from build123d import *

# Parameters (mm, degrees)
BASPROSKE_W         = 15
BASPROSKE_H         = 33
TOOTHCUT_DEPTH      = 50.020403915
TEETHCUTS_COUNT     = 20
TEETHCUTS_ANGLE     = 342
BORSKE_R            = 2
BORE_DEPTH          = 50.0000508
SKETCH1_W           = 29.7
SKETCH1_H           = 29.7
BOSS_EXTRUDE1_DEPTH = 20
SKETCH2_R           = 7.65
CUT_EXTRUDE1_DEPTH  = 35
FILLET2_R           = 1


with BuildPart() as part:
    # BasProSke → Base-Revolve (revolve)
    with BuildSketch(Plane(origin=(0, 0, 0), x_dir=(1, 0, 0), z_dir=(0, 1, 0)), mode=Mode.PRIVATE) as base_revolve_sk:
        with Locations((7.5, 16.5)):
            Rectangle(BASPROSKE_W, BASPROSKE_H)
    revolve(base_revolve_sk.sketch.rotate(Axis((-10, 0, 0), (1, 0, 0)), 180), axis=Axis((-10, 0, 0), (1, 0, 0)))

    # TooCutSke → ToothCut (cut, through all)
    with BuildSketch(Plane(origin=(0, 0, 0), x_dir=(0, 0, -1), z_dir=(1, 0, 0))):
        with BuildLine():
            ThreePointArc((1.489278925, 26.206717637), (0, 26.249), (-1.489278925, 26.206717637))
            ThreePointArc((-1.489278925, 26.206717637), (-2.448651415, 29.690511169), (-4.401620335, 32.730762038))
            ThreePointArc((-4.401620335, 32.730762038), (0, 33.0254), (4.401620335, 32.730762038))
            ThreePointArc((4.401620335, 32.730762038), (2.448651415, 29.690511169), (1.489278925, 26.206717637))
        make_face()
    toothcut = extrude(amount=TOOTHCUT_DEPTH, mode=Mode.SUBTRACT)

    # TeethCuts: ToothCut ×20 about axis
    teethcuts_axis = Axis((-10, 0, 0), (1, 0, 0))
    for i in range(1, TEETHCUTS_COUNT):
        add(toothcut.rotate(teethcuts_axis, i * TEETHCUTS_ANGLE / (TEETHCUTS_COUNT - 1)), mode=Mode.SUBTRACT)

    # BorSke → Bore (cut, symmetric)
    with BuildSketch(Plane(origin=(0, 0, 0), x_dir=(0, 0, -1), z_dir=(1, 0, 0))):
        with Locations(Location((0, 0, 0), (0, 0, 180))):
            Circle(BORSKE_R)
    extrude(amount=BORE_DEPTH, both=True, mode=Mode.SUBTRACT)

    # Sketch1 → Boss-Extrude1 (add)
    with BuildSketch(Plane(origin=(15, 0, 0), x_dir=(0, 0, -1), z_dir=(1, 0, 0))):
        Rectangle(SKETCH1_W, SKETCH1_H)
    extrude(amount=BOSS_EXTRUDE1_DEPTH)

    # Sketch2 → Cut-Extrude1 (cut)
    with BuildSketch(Plane.ZY):
        Circle(SKETCH2_R)
    extrude(amount=-CUT_EXTRUDE1_DEPTH, mode=Mode.SUBTRACT)

    # Fillet2
    fillet2_edges = [part.edges().sort_by_distance(p)[0] for p in [
        (25, 14.85, 14.85),
        (25, -14.85, 14.85),
        (25, -14.85, -14.85),
        (25, 14.85, -14.85),
        (35, 0, 14.85),
        (35, -14.85, 0),
        (35, 0, -14.85),
        (35, 14.85, 0),
    ]]
    fillet(fillet2_edges, radius=FILLET2_R)


solid = part.part
The listing builds one solid part. Answer for the finished solid, in the listing's coordinates (mm). A direction names the side the tool comes from. Round coordinates to 2 decimals unless told otherwise and drop trailing zeros. Order: outer loops, then holes, each group sorted by start corner. A loop starts at its lowest first (then second) coordinate and runs counter-clockwise, first axis right, second up. Notation, with made-up numbers: (-29.75, 85) - (5.25, 85) arc R16 cw to (5.25, 112) - close; hole circle Ø8 at (-31.5, 44). An arc over 180 degrees is marked (long way). Write item = value, one per line. Start each with the question number.
1) Straight lines are drawn through the part: L1, parallel to X at y = 27, z = -12; L2, parallel to Y at x = 24, z = 0; L3, parallel to Y at x = 27.5, z = -11. For each, find the intervals that lie inside material, in ascending order.
2) Section D-D, the plane z = 13 is taken. Write down the section's boundary in (x, y).
3) Section B-B, the plane x = 18 is taken. Write down the section's boundary in (y, z), plus the area to 3 significant figures.
4) For a pull along Z with two mould halves and no side action, classify faces 1 (the cylindrical face through (7.605, 5.151, -32.595)), 2 (the cylindrical face through (7.395, 25.494, 15.478)), 3 (the cylindrical face through (7.4, 29.72, -2.46)), 4 (the flat face through (35, 6, 6)) as released by +Z, released by -Z, zero draft, split by the parting line, or undercut.
5) For faces 5 (the flat face through (15, 0, 15)), 6 (the cylindrical face through (7.395, 28.929, -6.853)), 7 (the cylindrical face through (7.395, -19.463, -22.598)), 8 (the cylindrical face through (7.4, -19.38, 22.55)), determine the directions among +Z, -Z, +X, -X, +Y, -Y from which every point of the face is accessible in a straight line to the end or side of a thin tool.
6) Given pin 1 (4 mm diameter, centred on x = 26.5, y = 0.5, fed in from -Z); pin 2 (15 mm diameter, centred on x = 25, z = 1.5, fed in from -Y); pin 3 (4 mm diameter, centred on x = 15.5, y = 19.5, fed in from -Z); pin 4 (4 mm diameter, centred on x = 20.5, z = 17, fed in from +Y), each flat-ended and moving along its own axis, determine where each tip first touches the part or whether it passes through.
7) Section A-A, the plane y = 0 is taken. Write down the section's boundary in (x, z).
Results list:
q1.L1 = 0 to 15
q1.L2 = -14.85 to -7.65, 7.65 to 14.85
q1.L3 = -14.85 to 14.85
q2.outline = (0, -28.88) - (15, -28.88) - (15, -14.85) - (34, -14.85) arc R1 ccw to (35, -13.85) - (35, 13.85) arc R1 ccw to (34, 14.85) - (15, 14.85) - (15, 28.88) - (0, 28.88) - close
q3.outline = (-14.85, -13.85) arc R1 ccw to (-13.85, -14.85) - (13.85, -14.85) arc R1 ccw to (14.85, -13.85) - (14.85, 13.85) arc R1 ccw to (13.85, 14.85) - (-13.85, 14.85) arc R1 ccw to (-14.85, 13.85) - close; hole circle Ø15.3 at (0, 0)
q3.area = 697 mm^2
q4.face_1 = released by -Z
q4.face_2 = undercut
q4.face_3 = undercut
q4.face_4 = zero draft
q5.face_5 = +X
q5.face_6 = +X, -X
q5.face_7 = -Z, +X, -X
q5.face_8 = +Z, +X, -X
q6.pin_1 = -14.85
q6.pin_2 = -14.85
q6.pin_3 = -23.5
q6.pin_4 = through
q7.outline = (0, -26.25) - (15, -26.25) - (15, -14.85) - (34, -14.85) arc R1 ccw to (35, -13.85) - (35, -7.65) - (0, -7.65) - close; (0, 7.65) - (35, 7.65) - (35, 13.85) arc R1 ccw to (34, 14.85) - (15, 14.85) - (15, 26.25) - (0, 26.25) - close
